Geometry check sheet. Reference: drawing and pictorial views, mm from the part's lowest x, y, z. Round coordinates to 2 decimals unless told otherwise and drop trailing zeros. Order: outer loops, then holes, each group sorted by start corner. A loop starts at its lowest first (then second) coordinate and runs counter-clockwise, first axis right, second up.
(1) Go/stop test with a flat-tipped pin: pin 1 (2.5 mm diameter, centred on x = 3.15, y = 3.15, fed in from -Z). Record where the tip stops, or that it passes through.
(2) Sectioned sample at B-B (y = 3.15). Record the boundary of the cut face in (x, z), plus the area to 3 significant figures.
(3) Material ranges on line 1 along Y through (x, z) = (3.15, 0.8); line 2 along X through (y, z) = (4.5, 1.2), recorded low to high.
(4) Sectioned sample at A-A (x = 3.15). Record the boundary of the cut face in (y, z), plus the area to 3 significant figures.
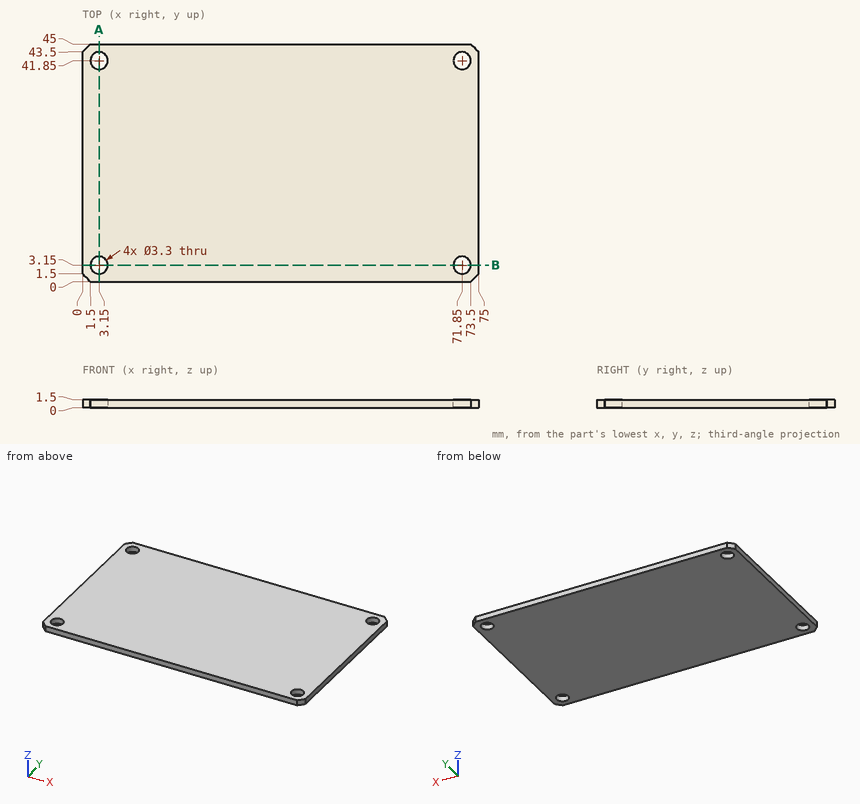
Answer below:
1. pin 1: passes through
2. outline: (0, 0) - (1.5, 0) - (1.5, 1.5) - (0, 1.5) - close; (4.8, 0) - (70.2, 0) - (70.2, 1.5) - (4.8, 1.5) - close; (73.5, 0) - (75, 0) - (75, 1.5) - (73.5, 1.5) - close
2. area: 103 mm2
3. line 1: y = 0 to 1.5, 4.8 to 40.2, 43.5 to 45
3. line 2: x = 0 to 2.2, 4.1 to 70.9, 72.8 to 75
4. outline: (0, 0) - (1.5, 0) - (1.5, 1.5) - (0, 1.5) - close; (4.8, 0) - (40.2, 0) - (40.2, 1.5) - (4.8, 1.5) - close; (43.5, 0) - (45, 0) - (45, 1.5) - (43.5, 1.5) - close
4. area: 57.6 mm2
